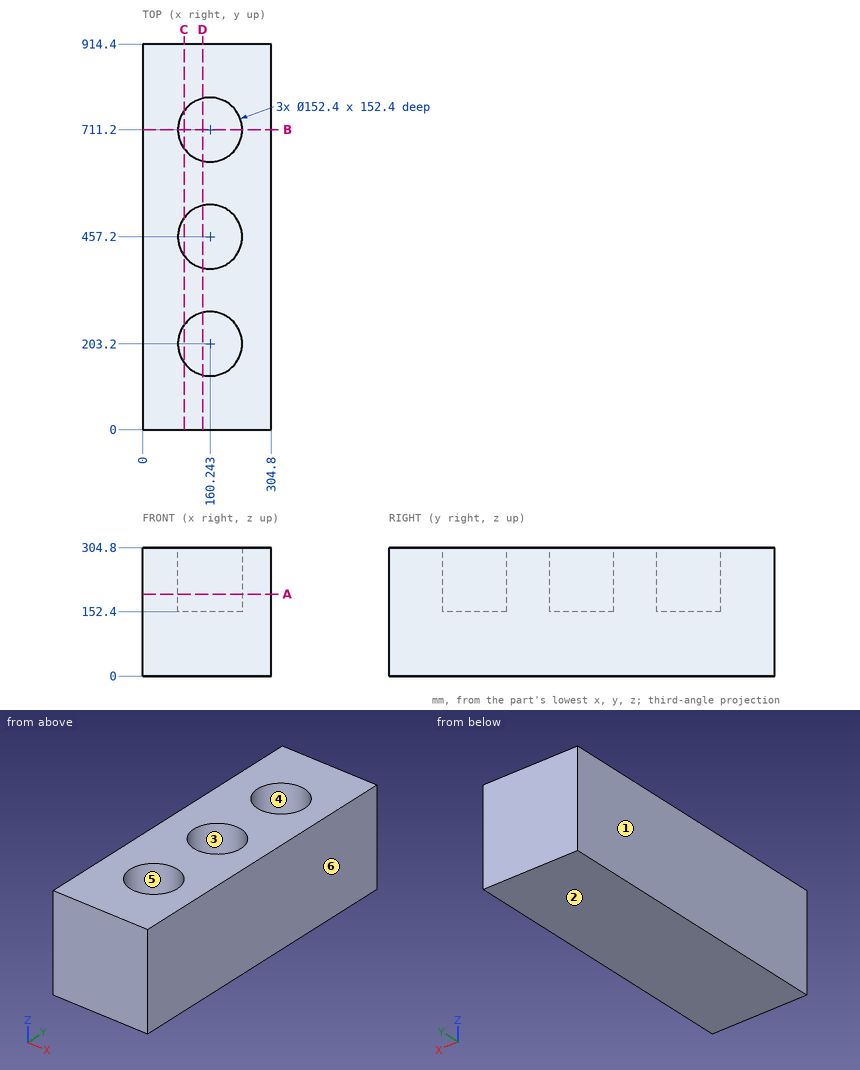
Here's the drawing with two shaded views (mm, measured from the low corner). I have some questions. A direction names the side the tool comes from. Coordinates: 2 decimals unless noted, no trailing zeros. Order: outer loops, then holes, each group sorted by start corner. A loop starts at its lowest first (then second) coordinate and runs counter-clockwise, first axis right, second up.
Q1. Please list where these lines run through material, in increasing order: L1, parallel to X at y = 457, z = 226; L2, parallel to Y at x = 189, z = 190 (1 decimal); L3, parallel to Y at x = 190.5, z = 178 (1 decimal).
Q2. Will this pin go through, and if not, where does the flat tip stop? pin 1 (5 mm diameter, centred on x = 183.5, y = 413.5, fed in from +Z).
Q3. Suppose I cut it at B-B on y = 711.2. Please give me the cut outline in (x, z), and give its area (3 significant figures).
Q4. Which directions (+Z, -Z, +X, -X, +Y, -Y) give clear straight access to the entire face, cutting with the end or side of a thin tool? Please do the marked faces 5 and 6.
Q5. Suppose I cut it at C-C on x = 98.5. Please give me the cut outline in (y, z), and give its area (3 significant figures).
Q6. Thinking about a two-plate mould opening in X: for the marked faces 1, 2, 3 and 4, which applies, released by +X, released by -X, zero draft, split by the parting line, or undercut?
Q7. Suppose I cut it at D-D on x = 142.5. Please give me the cut outline in (y, z) (1 decimal), and give its area (3 significant figures).
Q8. Suppose I cut it at A-A on z = 194. Please give me the cut outline in (x, y).
Answer:
1. L1: x = 0 to 84.04, 236.44 to 304.8
1. L2: y = 0 to 132.6, 273.8 to 386.6, 527.8 to 640.6, 781.8 to 914.4
1. L3: y = 0 to 133.3, 273.1 to 387.3, 527.1 to 641.3, 781.1 to 914.4
2. pin 1: stops at z = 152.4
3. outline: (0, 0) - (304.8, 0) - (304.8, 304.8) - (236.44, 304.8) - (236.44, 152.4) - (84.04, 152.4) - (84.04, 304.8) - (0, 304.8) - close
3. area: 69,700 mm2
4. face 5: +Z
4. face 6: +Z, -Z, +X, +Y, -Y
5. outline: (0, 0) - (914.4, 0) - (914.4, 304.8) - (755.86, 304.8) - (755.86, 152.4) - (666.54, 152.4) - (666.54, 304.8) - (501.86, 304.8) - (501.86, 152.4) - (412.54, 152.4) - (412.54, 304.8) - (247.86, 304.8) - (247.86, 152.4) - (158.54, 152.4) - (158.54, 304.8) - (0, 304.8) - close
5. area: 238,000 mm2
6. face 1: released by -X
6. face 2: zero draft
6. face 3: undercut
6. face 4: undercut
7. outline: (0, 0) - (914.4, 0) - (914.4, 304.8) - (785.3, 304.8) - (785.3, 152.4) - (637.1, 152.4) - (637.1, 304.8) - (531.3, 304.8) - (531.3, 152.4) - (383.1, 152.4) - (383.1, 304.8) - (277.3, 304.8) - (277.3, 152.4) - (129.1, 152.4) - (129.1, 304.8) - (0, 304.8) - close
7. area: 211,000 mm2
8. outline: (0, 0) - (304.8, 0) - (304.8, 914.4) - (0, 914.4) - close; hole circle Ø152.4 at (160.24, 203.2); hole circle Ø152.4 at (160.24, 457.2); hole circle Ø152.4 at (160.24, 711.2)
